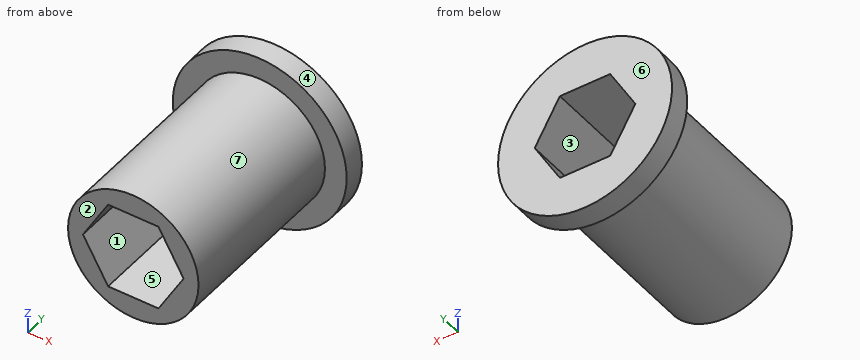
from build123d import *

# Parameters (mm, degrees)
SKETCH1_R           = 7.5
BOSS_EXTRUDE1_DEPTH = 21.05
SKETCH1_3_R         = 10
SKETCH1_3_R_2       = 7.5
BOSS_EXTRUDE2_DEPTH = 2.54


with BuildPart() as part:
    # Sketch1 → Boss-Extrude1 (new body)
    with BuildSketch(Plane(origin=(0, 0, 0), x_dir=(1, 0, 0), z_dir=(0, 1, 0))):
        Circle(SKETCH1_R)
        Polygon((-5.787936449, 0), (-2.893968224, -5.0125), (2.893968224, -5.0125), (5.787936449, 0), (2.893968224, 5.0125), (-2.893968224, 5.0125), align=None, mode=Mode.SUBTRACT)
    extrude(amount=-BOSS_EXTRUDE1_DEPTH)

    # Sketch1_3 → Boss-Extrude2 (add)
    with BuildSketch(Plane(origin=(0, 0, 0), x_dir=(1, 0, 0), z_dir=(0, 1, 0))):
        Circle(SKETCH1_3_R)
        Circle(SKETCH1_3_R_2, mode=Mode.SUBTRACT)
        Circle(SKETCH1_3_R_2)
        Polygon((-5.787936449, 0), (-2.893968224, -5.0125), (2.893968224, -5.0125), (5.787936449, 0), (2.893968224, 5.0125), (-2.893968224, 5.0125), align=None, mode=Mode.SUBTRACT)
    extrude(amount=BOSS_EXTRUDE2_DEPTH)


solid = part.part
The listing builds one solid part. Answer for the finished solid, in the listing's coordinates (mm). Face numbers are marked on the shaded views. A direction names the side the tool comes from. Coordinates: 2 decimals unless noted, no trailing zeros. Order: outer loops, then holes, each group sorted by start corner. A loop starts at its lowest first (then second) coordinate and runs counter-clockwise, first axis right, second up.
Q1. A cutting plane is placed at B-B, the plane z = 2.25. Write down the section's boundary in (x, y), and give its area (3 significant figures).
Q2. Given P1, Ø5, axis at x = -3.5, y = -1, coming from the +Z side; P2, Ø1.7, axis at x = 1.5, y = -3.5, coming from the +Z side; P3, Ø12, axis at y = -8.5, z = 5, coming from the +X side, each flat-ended and moving along its own axis, determine where each tip first touches the part or whether it passes through.
Q3. Which of the six approach directions +Z, -Z, +X, -X, +Y, -Y give full straight-line access (tool end or side, diameter ignored) to the marked faces 5, 6 and 7?
Q4. Consider line 1 (X direction, y = -4.5, z = -3.25); line 2 (Z direction, x = -4, y = 1); line 3 (X direction, y = -15, z = -1.25). Determine where each line is inside the solid, lowest interval first.
Q5. For a pull along Z with two mould halves and no side action, classify the marked faces 1, 2, 3 and 4 as pulls with the +Z half, pulls with the -Z half, needs draft (parallel to the pull), parting line crosses it, or undercut.
Q6. A cutting plane is placed at D-D, the plane z = -6. Write down the section's boundary in (x, y), and give its area (3 significant figures).
Q7. A cutting plane is placed at A-A, the plane x = 0. Write down the section's boundary in (y, z), and give its area (3 significant figures).
Q8. A cutting plane is placed at C-C, the plane y = -3.5. Write down the section's boundary in (x, z), and give its area (3 significant figures).
Answers follow:
1. outline: (-9.74, 0) - (-7.15, 0) - (-7.15, -21.05) - (-4.49, -21.05) - (-4.49, 2.54) - (-9.74, 2.54) - close; (4.49, -21.05) - (7.15, -21.05) - (7.15, 0) - (9.74, 0) - (9.74, 2.54) - (4.49, 2.54) - close
1. area: 139 mm2
2. P1: stops at z = 9.93
2. P2: stops at z = 7.47
2. P3: stops at x = 7.5
3. face 5: +Y, -Y
3. face 6: +Z, -Z, +X, -X, +Y
3. face 7: -Y
4. line 1: x = -6.76 to -3.91, 3.91 to 6.76
4. line 2: z = -9.17 to -3.1, 3.1 to 9.17
4. line 3: x = -7.4 to -5.07, 5.07 to 7.4
5. face 1: undercut
5. face 2: needs draft
5. face 3: undercut
5. face 4: parting line crosses it
6. outline: (-8, 0) - (-4.5, 0) - (-4.5, -21.05) - (4.5, -21.05) - (4.5, 0) - (8, 0) - (8, 2.54) - (-8, 2.54) - close
6. area: 230 mm2
7. outline: (-21.05, -7.5) - (0, -7.5) - (0, -10) - (2.54, -10) - (2.54, -5.01) - (-21.05, -5.01) - close; (-21.05, 5.01) - (2.54, 5.01) - (2.54, 10) - (0, 10) - (0, 7.5) - (-21.05, 7.5) - close
7. area: 130 mm2
8. outline: circle Ø15 at (0, 0); hole (-5.79, 0) - (-2.89, -5.01) - (2.89, -5.01) - (5.79, 0) - (2.89, 5.01) - (-2.89, 5.01) - close
8. area: 89.7 mm2
